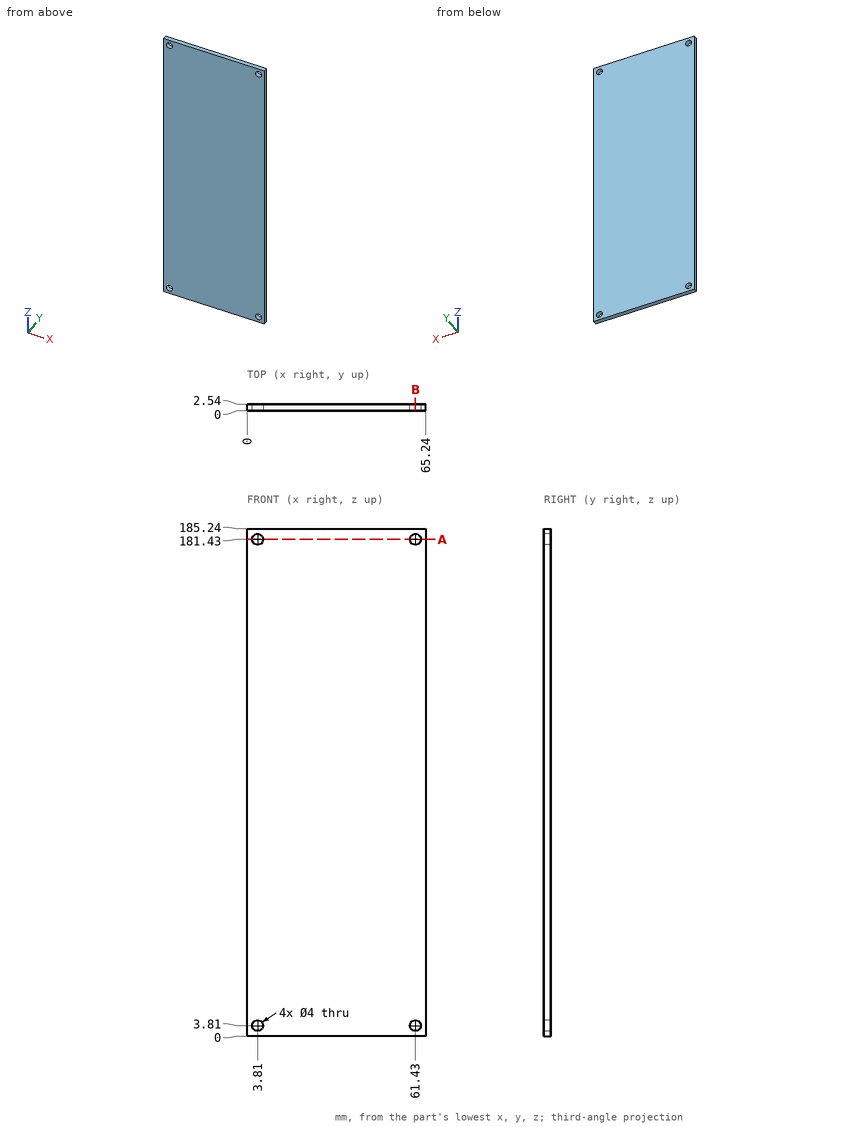
Geometry: see drawing. Coordinates: mm, zero at the bounding-box minimum. Coordinates: 2 decimals unless noted, no trailing zeros. Order: outer loops, then holes, each group sorted by start corner. A loop starts at its lowest first (then second) coordinate and runs counter-clockwise, first axis right, second up. Notation, with made-up numbers: M 28.25,6.5 L 62.25,6.5 A13 ccw 62.25,29.5 Z; hole C 78,79.5 d2. An arc over 180 degrees is marked long. Write item = value, one per line. Start each with the question number.
(1) Section B-B on x = 61.43. Output: boundary loops of the cut face in (y, z).
(2) First-contact query: P1, Ø3.5, axis at x = 61.43, z = 181.43, coming from the -Y side (1 decimal). Flat tip, straight axial feed; report the tip coordinate or a pass-through.
(3) Section A-A on z = 181.43. Output: boundary loops of the cut face in (x, y), and give its area (3 significant figures).
(4) Line query: line 1 along Z through (x, y) = (61.43, 1.8); line 2 along X through (y, z) = (2.05, 181.43). Output: solid intervals per line, ascending. Write a range as [from, to].
Result set:
q1.outline = M 0,0 L 2.54,0 L 2.54,1.81 L 0,1.81 Z; M 0,5.81 L 2.54,5.81 L 2.54,179.43 L 0,179.43 Z; M 0,183.43 L 2.54,183.43 L 2.54,185.24 L 0,185.24 Z
q2.P1 = through
q3.outline = M 0,0 L 1.81,0 L 1.81,2.54 L 0,2.54 Z; M 5.81,0 L 59.43,0 L 59.43,2.54 L 5.81,2.54 Z; M 63.43,0 L 65.24,0 L 65.24,2.54 L 63.43,2.54 Z
q3.area = 145 mm²
q4.line_1 = [0, 1.81], [5.81, 179.43], [183.43, 185.24]
q4.line_2 = [0, 1.81], [5.81, 59.43], [63.43, 65.24]
